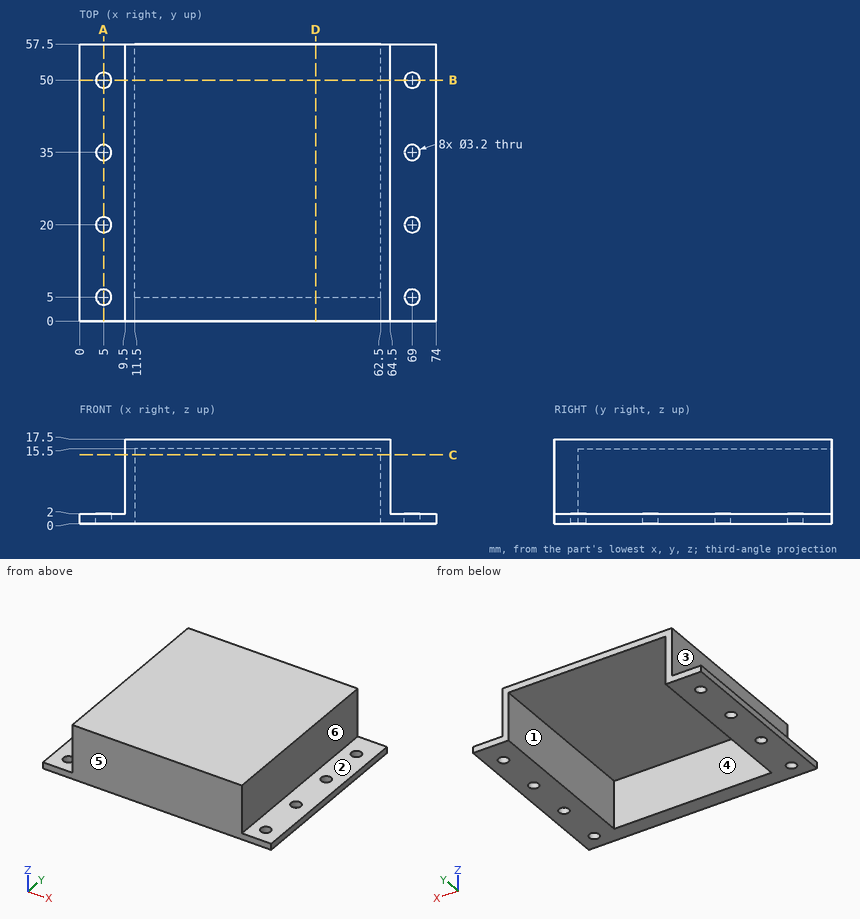
Here's the drawing with two shaded views (mm, measured from the low corner). I have some questions. A direction names the side the tool comes from. Coordinates: 2 decimals unless noted, no trailing zeros. Loops run counter-clockwise (first coordinate to the right, second up) from the corner with the lowest first, then second, coordinate; pieces in that order, holes last. Notation, with made-up numbers: M -23,24 L 16,24 A20 ccw 16,34 Z; hole C 47,-26 d4. An arc over 180 degrees is marked long. Return JSON: item names as keys, results as strings. Group by question number.
Item 1: Imagine slicing it at C-C (z = 14.25). Please give me the cut outline in (x, y), and give its area (3 significant figures).
Item 2: I'm going to push flat-ended pins straight in: pin 1 Ø4.5 at (y, z) = (19, 9.5) entering from -X; pin 2 Ø5 at (x, y) = (5, 20) entering from +Z; pin 3 Ø8 at (x, z) = (26, 11) entering from +Y. Where does each tip first touch, or does it pass through?
Item 3: Imagine slicing it at D-D (x = 49). Please give me the cut outline in (y, z), and give its area (4 significant figures).
Item 4: Imagine slicing it at B-B (y = 50). Please give me the cut outline in (x, z), and give its area (3 significant figures).
Item 5: If I drill on L1, parallel to Y at x = 5, z = 1.25; L2, parallel to X at y = 11, z = 7.5; L3, parallel to Z at x = 16.5, y = 36, over which ranges is the centre line in solid material (lowest first)? Write a range as from..to.
Item 6: On a 3-axis mill with a long thin cutter (end or side, diameter ignored), from which of +Z, -Z, +X, -X, +Y, -Y can I reach the whole of each face in a straight line? I mean the marked faces 1, 2 and 3. Say none if no direction works.
Item 7: Thinking about a two-plate mould opening in X: for the marked faces 4, 5 and 6, which applies, released by +X, released by -X, zero draft, split by the parting line, or undercut?
Item 8: Imagine slicing it at A-A (x = 5). Please give me the cut outline in (y, z).
Verdict:
{
 "1": {"outline": "M 9.5,0 L 64.5,0 L 64.5,57.5 L 62.5,57.5 L 62.5,5 L 11.5,5 L 11.5,57.5 L 9.5,57.5 Z", "area": "485 mm^2"},
 "2": {"pin 1": "stops at x = 9.5", "pin 2": "stops at z = 2", "pin 3": "stops at y = 5"},
 "3": {"outline": "M 0,0 L 5,0 L 5,15.5 L 57.5,15.5 L 57.5,17.5 L 0,17.5 Z", "area": "192.5 mm^2"},
 "4": {"outline": "M 0,0 L 3.4,0 L 3.4,2 L 0,2 Z; M 6.6,0 L 11.5,0 L 11.5,15.5 L 62.5,15.5 L 62.5,0 L 67.4,0 L 67.4,2 L 64.5,2 L 64.5,17.5 L 9.5,17.5 L 9.5,2 L 6.6,2 Z; M 70.6,0 L 74,0 L 74,2 L 70.6,2 Z", "area": "197 mm^2"},
 "5": {"L1": "y = 0..3.4, 6.6..18.4, 21.6..33.4, 36.6..48.4, 51.6..57.5", "L2": "x = 9.5..11.5, 62.5..64.5", "L3": "z = 15.5..17.5"},
 "6": {"face 1": "-Z, +Y", "face 2": "+Z, +X, +Y, -Y", "face 3": "+Z, -X, +Y, -Y"},
 "7": {"face 4": "undercut", "face 5": "zero draft", "face 6": "released by +X"},
 "8": {"outline": "M 0,0 L 3.4,0 L 3.4,2 L 0,2 Z; M 6.6,0 L 18.4,0 L 18.4,2 L 6.6,2 Z; M 21.6,0 L 33.4,0 L 33.4,2 L 21.6,2 Z; M 36.6,0 L 48.4,0 L 48.4,2 L 36.6,2 Z; M 51.6,0 L 57.5,0 L 57.5,2 L 51.6,2 Z"}
}
